Autodesk Inventor part; units mm, degrees
ref_plane "Start plane" through (0, 0, 0) normal (0, 0, 1) x (1, 0, 0)
ref_plane "End plane" through (0, 0, 609.6) normal (0, 0, 1) x (1, 0, 0)
ref_plane "YZ Plane" through (0, 0, 0) normal (1, 0, 0) x (0, 1, 0)
ref_plane "Start plane" through (0, 0, 0) normal (0, 0, 1) x (1, 0, 0)
ref_plane "End plane" through (0, 0, 609.6) normal (0, 0, 1) x (1, 0, 0)
sketch "Sketch" plane through (0, 0, 0) normal (0, 0, 1) x (1, 0, 0)
  line L0 (25.4, 0) -> (0, 0)
  line L1 (0, 0) -> (0, 25.4)
  line L2 (0, 25.4) -> (1.651, 25.4)
  line L3 (3.175, 23.876) -> (3.175, 6.477)
  line L4 (6.477, 3.175) -> (23.876, 3.175)
  line L5 (25.4, 1.651) -> (25.4, 0)
  line L6 (0, -11.0414) -> (0, 31.5385) construction
  line L7 (-11.0414, 0) -> (31.5385, 0) construction
  arc A0 (3.175, 6.477) -> (6.477, 3.175) centre (6.477, 6.477) ccw
  arc A1 (3.175, 23.876) -> (1.651, 25.4) centre (1.651, 23.876) ccw
  arc A2 (25.4, 1.651) -> (23.876, 3.175) centre (23.876, 1.651) ccw
  line L8 (0, 40.0545) -> (0, -19.5574) construction
  line L9 (-19.5574, 0) -> (40.0545, 0) construction
  point P0 (3.175, 25.4)
  point P1 (3.175, 3.175)
  point P2 (25.4, 3.175)
  dimension "d0" = 25.4
  dimension "d1" = 25.4
  dimension "d2" = 3.175
  dimension "d3" = 3.175
  dimension "d10" = 0
  dimension "d11" = 0
  dimension "d14" = 3.302
  dimension "d15" = 1.524
extrude "Body" add sketch "Sketch" along normal up to surface (609.6 mm away) from surface at 0
sketch "Sketch3" plane through (0, 0, 0) normal (0, 0, 1) x (1, 0, 0)
  line L0 (0, 0) -> (10, 0)
ref_plane "Work Plane3" through (0, 0, 0) normal (0, -1, 0) x (1, 0, 0)
sketch "Sketch4" plane through (0, 0, 0) normal (0, -1, 0) x (1, 0, 0)
  line L0 (-2, 0) -> (12, 0)
  line L1 (-2, 609.6) -> (12, 609.6)
  dimension "d17" = 609.6
sketch "Sketch12" plane through (0, 0, 0) normal (0, -1, 0) x (1, 0, 0)
  line L0 (25.4, 0) -> (25.4, 609.6)
  line L1 (25.4, 19.05) -> (12.7, 19.05)
  line L2 (12.7, 19.05) -> (12.7, 29.05)
  line L3 (12.7, 29.05) -> (25.4, 29.05)
  line L4 (25.4, 29.05) -> (25.4, 19.05)
  line L5 (25.4, 0) -> (0, 0)
  arc A0 (12.7, 29.05) -> (12.7, 19.05) centre (16.0166, 24.05) ccw
  point P0 (25.4, 29.05)
  dimension "d47" = 12.7
  dimension "d48" = 10
  dimension "d49" = 19.05
  dimension "d50" = 6
extrude "Extrusion6" cut sketch "Sketch12" against normal through all
equation "\"d0\" = G_H"
equation "\"d1\" = G_H"
equation "\"d2\" = G_T"
equation "\"d3\" = G_T"
equation "\"d14\" = G_IR"
equation "\"d15\" = G_ER"
equation "\"d4\" = G_L"
equation "\"d47\" = axle_inset_up"
equation "\"d49\" = axle_inset_fwd"
equation "\"G_H\" = 25.4"
equation "\"G_T\" = 3.175"
equation "\"G_ER\" = 1.524"
equation "\"G_IR\" = 3.302"
equation "\"G_L\" = d17"
equation "\"ex\" = 0"
equation "\"G_OFFSET_START\" = 0"
equation "\"G_OFFSET_END\" = 0"
equation "\"d13\" = G_OFFSET_END + B_L"
equation "\"B_L\" = 609.6"
equation "\"axle_inset_up\" = 12.7"
equation "\"axle_inset_fwd\" = 19.05"
properties part number "AISC - L 1 x 1 x 1/8 - 24" material "Steel, Mild"
Read the model definition and answer for the solid it produces. Units are mm, in the model's axes. A direction names the side the tool comes from. Coordinates: 2 decimals unless noted, no trailing zeros. Write each loop counter-clockwise with the first axis right and the second up, starting at its lowest first coordinate (ties: lowest second). Pieces come first, ordered by that corner, then holes. Notation, with made-up numbers: M 12,-15.5 L 46,-15.5 A27 ccw 46,14.5 Z; hole C 7,11.5 d11. An arc over 180 degrees is marked long. Use a Markdown table: item, result.
Q1. Straight lines are drawn through the part: L1, parallel to Z at x = 20.75, y = 2; L2, parallel to Y at x = 12.25, z = 193.5 (3 decimals). For each, find the intervals that lie inside material, in ascending order. Write a range as [from, to].
Answer block:
| item | result |
|---|---|
| L1 | z = [0, 19.05], [29.05, 609.6] |
| L2 | y = [0, 3.175] |
Q2. The part is cut by section B-B, the plane z = 150. Write down the section's boundary in (x, y) (3 decimals), then the cut area to 3 significant figures.
Answer block:
| item | result |
|---|---|
| outline | M 0,0 L 25.4,0 L 25.4,1.651 A1.524 ccw 23.876,3.175 L 6.477,3.175 A3.302 cw 3.175,6.477 L 3.175,23.876 A1.524 ccw 1.651,25.4 L 0,25.4 Z |
| area | 153 mm2 |
Q3. Each of these flat-tipped pins is pushed along its axis until it touches: pin 1 Ø4 at (x, y) = (7, 9.5) entering from +Z; pin 2 Ø8.5 at (x, z) = (17.5, 440) entering from +Y (3 decimals); pin 3 Ø14 at (y, z) = (11, 307) entering from +X; pin 4 Ø6 at (y, z) = (8.5, 75) entering from +X. Where does it stop, or does it pass through?
Answer block:
| item | result |
|---|---|
| pin 1 | passes through |
| pin 2 | stops at y = 3.175 |
| pin 3 | stops at x = 4.29 |
| pin 4 | stops at x = 3.32 |
Q4. The part is cut by section A-A, the plane x = 20. Write down the section's boundary in (y, z) (3 decimals), then the cut area to 3 significant figures.
Answer block:
| item | result |
|---|---|
| outline | M 0,0 L 3.175,0 L 3.175,19.05 L 0,19.05 Z; M 0,29.05 L 3.175,29.05 L 3.175,609.6 L 0,609.6 Z |
| area | 1,900 mm2 |
Q5. Which of the six approach directions +Z, -Z, +X, -X, +Y, -Y give full straight-line access (tool end or side, diameter ignored) to faces 1 (the face through (3.175, 15, 301)), 2 (the face through (0, 13, 301))?
Answer block:
| item | result |
|---|---|
| face 1 | +Z, -Z, +X, +Y |
| face 2 | +Z, -Z, -X, +Y, -Y |
Q6. The part is cut by section C-C, the plane y = 18.25. Write down the section's boundary in (x, z) (3 decimals), then the cut area to 3 significant figures.
Answer block:
| item | result |
|---|---|
| outline | M 0,0 L 3.175,0 L 3.175,609.6 L 0,609.6 Z |
| area | 1,940 mm2 |
